Check sheet for the modelled part. Datum: model origin and axes. Units: mm. Face numbers are marked on the shaded views. A direction names the side the tool comes from. Round coordinates to 2 decimals unless told otherwise and drop trailing zeros. Loops run counter-clockwise (first coordinate to the right, second up) from the corner with the lowest first, then second, coordinate; pieces in that order, holes last. Notation, with made-up numbers: (-21, -5) - (27, -5) arc R28 ccw to (27, 22) - close; hole circle Ø5 at (-35, 63). An arc over 180 degrees is marked (long way). Answer in a Markdown table with one row per item. Add a question column.
(1) Thickness scan on line 1 along X through (y, z) = (-3, 2); line 2 along Y through (x, z) = (0, 2.95) (3 decimals); line 3 along X through (y, z) = (-1.25, 3). Record the ranges inside material, lowest first.
(2) Mould release check, pull along Z, two halves, no side actions. Record for the marked faces 1, 2 and 3: +Z half, -Z half, draft (parallel to the pull), parting line (faces both ways), or undercut.
(3) Cross-section at D-D on x = -9. Enter the section's corners in (y, z) (3 decimals).
(4) Access from +Z, -Z, +X, -X, +Y, -Y to the whole of each face (thin tool, end or side, straight path). Record for the marked faces 4, 5 and 6.
(5) Gauge pin test, flat ends, axial feed: pin 1 (3.5 mm diameter, centred on y = -3.5, z = 3, fed in from +X); pin 2 (1.5 mm diameter, centred on y = -5.5, z = 5, fed in from -X); pin 3 (2.5 mm diameter, centred on y = -3, z = 2.5, fed in from -X); pin 4 (1.8 mm diameter, centred on x = 9.5, y = -11, fed in from -Z). Record the tip position at first contact, or that the pin passes through.
(6) Cross-section at C-C on y = -3.25. Enter the section's corners in (x, z) (3 decimals), then the cut area to 3 significant figures.
from build123d import *

# Parameters (mm, degrees)
SKETCH1_R                     = 19.05
SKETCH1_R_2                   = 0.5
BOSS_EXTRUDE1_DEPTH           = 6.35
M3_CLEARANCE_HOLE1_D          = 3.2
M3_CLEARANCE_HOLE1_DEPTH      = 29.72
M3_CLEARANCE_HOLE1_TIP        = 0.96137699
SKETCH4_W                     = 38.1
SKETCH4_H                     = 0.25
CUT_EXTRUDE1_DEPTH            = 28.679008291
CBORE_FOR_M2_SHCS1_AT_2_COUNT = 2
CBORE_FOR_M2_SHCS1_AT_2_PITCH = 18
CUT_EXTRUDE2_DEPTH            = 15
FILLET1_R                     = 2.38125
SKETCH12_W                    = 55.779861043
SKETCH12_H                    = 26.707675132
CUT_EXTRUDE3_DEPTH            = 28.678726197
SKETCH13_W                    = 5
SKETCH13_H                    = 3
CUT_EXTRUDE4_DEPTH            = 5
FILLET4_R                     = 0.5


with BuildPart() as part:
    # Sketch1 → Boss-Extrude1 (new body)
    with BuildSketch(Plane.XY):
        Circle(SKETCH1_R)
        with Locations((-6.049187445, 3.4925)):
            Circle(SKETCH1_R_2, mode=Mode.SUBTRACT)
        with Locations((6.049187445, 3.4925)):
            Circle(SKETCH1_R_2, mode=Mode.SUBTRACT)
        with Locations((0, -6.985)):
            Circle(SKETCH1_R_2, mode=Mode.SUBTRACT)
        with BuildLine():
            ThreePointArc((2.286, 0), (0, 2.286), (-2.286, 0))
            ThreePointArc((-2.286, 0), (0, -2.286), (2.286, 0))
        make_face(mode=Mode.SUBTRACT)
    extrude(amount=BOSS_EXTRUDE1_DEPTH)

    # M3 Clearance Hole1
    with Locations(Plane(origin=(-15.665967818, 20.219646462, 6.35), x_dir=(1, 0, 0), z_dir=(0, 0, 1))):
        with Locations((15.665967818, -5.554949625), (2.965967818, -27.551994881), (28.365967818, -27.551994881)):
            Hole(M3_CLEARANCE_HOLE1_D / 2, depth=M3_CLEARANCE_HOLE1_DEPTH)
            with Locations((0, 0, -(M3_CLEARANCE_HOLE1_DEPTH + M3_CLEARANCE_HOLE1_TIP / 2))):  # 118° drill point
                Cone(0, M3_CLEARANCE_HOLE1_D / 2, M3_CLEARANCE_HOLE1_TIP, mode=Mode.SUBTRACT)

    # Sketch4 → Cut-Extrude1 (cut, through all)
    with BuildSketch(Plane(origin=(0, 0, 0), x_dir=(-1, 0, 0), z_dir=(0, 0, -1))):
        Rectangle(SKETCH4_W, SKETCH4_H)
    extrude(amount=-CUT_EXTRUDE1_DEPTH, mode=Mode.SUBTRACT)


with BuildPart() as cut_extrude1_piece_1:
    # of the separate pieces the step leaves, piece 1, a body of its own (cut_extrude1_pieces)
    add(part.part.solids().sort_by_distance((19.049589891, 0.125, 0))[0])


with BuildPart() as cut_extrude1_piece_2:
    # of the separate pieces the step leaves, piece 2, a body of its own (cut_extrude1_pieces)
    add(part.part.solids().sort_by_distance((-19.049589891, -0.125, 0))[0])


with BuildPart() as cbore_for_m2_shcs1_tool:
    # Sketch9 → CBORE for M2 SHCS1 (revolve)
    with BuildSketch(Plane(origin=(-9, 19.05, 3.175), x_dir=(0, 0, 1), z_dir=(1, 0, 0))):
        Polygon((0, 0), (0, 38.1), (1.1, 38.1), (1.1, 2), (2.2, 2), (2.2, 0), align=None)
    cbore_for_m2_shcs1 = revolve(axis=Axis((-9, 25.4, 3.175), (0, -1, 0)))


with BuildPart() as cut_extrude1_piece_1_1:
    add(cut_extrude1_piece_1.part)

    # CBORE for M2 SHCS1: cut by cbore_for_m2_shcs1_tool
    add(cbore_for_m2_shcs1_tool.part, mode=Mode.SUBTRACT)


with BuildPart() as cut_extrude1_piece_2_1:
    add(cut_extrude1_piece_2.part)

    # CBORE for M2 SHCS1: cut by cbore_for_m2_shcs1_tool
    add(cbore_for_m2_shcs1_tool.part, mode=Mode.SUBTRACT)


with BuildPart() as cbore_for_m2_shcs1_at_2_tool:
    # CBORE for M2 SHCS1 at 2: CBORE for M2 SHCS1 ×2
    with Locations(*[(i * CBORE_FOR_M2_SHCS1_AT_2_PITCH, 0, 0) for i in range(1, CBORE_FOR_M2_SHCS1_AT_2_COUNT)]):
        add(cbore_for_m2_shcs1)


with BuildPart() as cut_extrude1_piece_1_2:
    add(cut_extrude1_piece_1_1.part)

    # CBORE for M2 SHCS1 at 2: cut by cbore_for_m2_shcs1_at_2_tool
    add(cbore_for_m2_shcs1_at_2_tool.part, mode=Mode.SUBTRACT)

    # Sketch12 → Cut-Extrude3 (cut, through all)
    with BuildSketch(Plane.XY):
        with Locations((0.042756797, 13.353837566)):
            Rectangle(SKETCH12_W, SKETCH12_H)
    extrude(amount=CUT_EXTRUDE3_DEPTH, mode=Mode.SUBTRACT)


with BuildPart() as cut_extrude1_piece_2_2:
    add(cut_extrude1_piece_2_1.part)

    # CBORE for M2 SHCS1 at 2: cut by cbore_for_m2_shcs1_at_2_tool
    add(cbore_for_m2_shcs1_at_2_tool.part, mode=Mode.SUBTRACT)

    # Sketch11 → Cut-Extrude2 (cut)
    with BuildSketch(Plane.XZ.offset(19.05)):
        Polygon((-10.154700538, 5.175), (-11.309401077, 3.175), (-10.154700538, 1.175), (-7.845299462, 1.175), (-6.690598923, 3.175), (-7.845299462, 5.175), align=None)
        Polygon((7.845299462, 5.175), (6.690598923, 3.175), (7.845299462, 1.175), (10.154700538, 1.175), (11.309401077, 3.175), (10.154700538, 5.175), align=None)
    extrude(amount=-CUT_EXTRUDE2_DEPTH, mode=Mode.SUBTRACT)

    # Fillet1
    fillet1_edges = [cut_extrude1_piece_2_2.edges().sort_by_distance(p)[0] for p in [
        (-0.5, -6.985, 0),
        (-0.5, -6.985, 6.35),
    ]]
    fillet(fillet1_edges, radius=FILLET1_R)

    # Sketch13 → Cut-Extrude4 (cut)
    with BuildSketch(Plane(origin=(0, -0.125, 0), x_dir=(1, 0, 0), z_dir=(0, 1, 0))):
        with Locations((-15.5, -3.175)):
            Rectangle(SKETCH13_W, SKETCH13_H)
        with Locations((15.5, -3.175)):
            Rectangle(SKETCH13_W, SKETCH13_H)
    extrude(amount=-CUT_EXTRUDE4_DEPTH, mode=Mode.SUBTRACT)

    # Fillet4
    fillet4_edges = [cut_extrude1_piece_2_2.edges().sort_by_distance(p)[0] for p in [
        (18, -0.125, 3.175),
        (15.5, -0.125, 1.675),
        (13, -0.125, 3.175),
        (15.5, -0.125, 4.675),
        (-15.5, -0.125, 1.675),
        (-18, -0.125, 3.175),
        (-15.5, -0.125, 4.675),
        (-13, -0.125, 3.175),
    ]]
    fillet(fillet4_edges, radius=FILLET4_R)


solid = cut_extrude1_piece_2_2.part
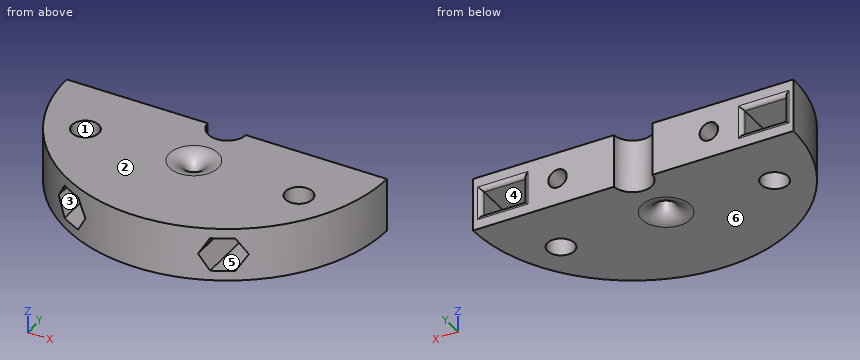
Answers:
| question | item | result |
|---|---|---|
| 1 | line 1 | x = -18.81 to -18, -13 to 13, 18 to 18.81 |
| 1 | line 2 | y = -19.05 to -7.485, -6.485 to -2.286 |
| 1 | line 3 | x = -19.01 to -18, -13 to -10.09, -7.91 to -1.91, 1.91 to 7.91, 10.09 to 13, 18 to 19.01 |
| 2 | face 1 | draft |
| 2 | face 2 | +Z half |
| 2 | face 3 | undercut |
| 3 | outline | (-16.79, 0) - (-0.125, 0) - (-0.125, 2.075) - (-4.05, 2.075) - (-4.05, 1.175) - (-16.79, 1.175) - close; (-16.79, 5.175) - (-4.05, 5.175) - (-4.05, 4.275) - (-0.125, 4.275) - (-0.125, 6.35) - (-16.79, 6.35) - close |
| 4 | face 4 | +Y |
| 4 | face 5 | -Y |
| 4 | face 6 | -Z, +X, -X, +Y, -Y |
| 5 | pin 1 | stops at x = 18.97 |
| 5 | pin 2 | stops at x = -18.45 |
| 5 | pin 3 | stops at x = -18.97 |
| 5 | pin 4 | stops at z = 0 |
| 6 | outline | (-18.771, 0) - (18.771, 0) - (18.771, 6.35) - (-18.771, 6.35) - close; hole (-18, 1.675) - (-13, 1.675) - (-13, 4.675) - (-18, 4.675) - close; hole circle Ø2.2 at (-9, 3.175); hole circle Ø2.2 at (9, 3.175); hole (13, 1.675) - (18, 1.675) - (18, 4.675) - (13, 4.675) - close |
| 6 | area | 201 mm^2 |
